Could you check a few things on this model? Use its own coordinates, in mm. A direction names the side the tool comes from. Give positions to 0.01 mm unless a question says otherwise; leave off trailing zeros. Loops run counter-clockwise (first coordinate to the right, second up) from the corner with the lowest first, then second, coordinate; pieces in that order, holes last. Notation, with made-up numbers: M 68,16.5 L 75,16.5 A29 cw 75,50.5 Z; hole C 24,47.25 d10. An arc over 180 degrees is marked long. Use CSV: the item, a comma, the result in double quotes.
```python
from build123d import *

# Parameters (mm, degrees)
SKETCH1_W            = 195
SKETCH1_H            = 145
BOSS_EXTRUDE1_DEPTH  = 5
SKETCH2_W            = 63.6
SKETCH2_H            = 2
SKETCH2_W_2          = 63.5
BOSS_EXTRUDE2_DEPTH  = 9.5
SKETCH4_W            = 8
SKETCH4_H            = 8
BOSS_EXTRUDE3_DEPTH  = 30
SKETCH3_W            = 2
SKETCH3_H            = 19
BOSS_EXTRUDE11_DEPTH = 12.6
SKETCH8_W            = 14
SKETCH8_H            = 14
SKETCH8_W_2          = 8
SKETCH8_H_2          = 8
BOSS_EXTRUDE12_DEPTH = 2
FILLET2_R            = 10
FILLET3_R            = 3


with BuildPart() as part:
    # Sketch1 → Boss-Extrude1 (new body)
    with BuildSketch(Plane(origin=(0, 0, 0), x_dir=(1, 0, 0), z_dir=(0, 1, 0))):
        Rectangle(SKETCH1_W, SKETCH1_H)
    extrude(amount=BOSS_EXTRUDE1_DEPTH)

    # Sketch2 → Boss-Extrude2 (add)
    with BuildSketch(Plane(origin=(0, 5, 0), x_dir=(1, 0, 0), z_dir=(0, 1, 0))):
        Polygon((-82.5, -57.5), (-82.5, -3.6), (-70, -3.6), (-70, -1.6), (-84.5, -1.6), (-84.5, -59.5), (84.5, -59.5), (84.5, -1.6), (70, -1.6), (70, -3.6), (82.5, -3.6), (82.5, -57.5), align=None)
        with Locations((-33.9, -2.6)):
            Rectangle(SKETCH2_W, SKETCH2_H)
        with Locations((33.95, -2.6)):
            Rectangle(SKETCH2_W_2, SKETCH2_H)
    extrude(amount=BOSS_EXTRUDE2_DEPTH)

    # Sketch4 → Boss-Extrude3 (add)
    with BuildSketch(Plane(origin=(0, 5, 0), x_dir=(1, 0, 0), z_dir=(0, 1, 0))):
        with Locations((-90.5, -65.5)):
            Rectangle(SKETCH4_W, SKETCH4_H)
        with Locations((90.5, -65.5)):
            Rectangle(SKETCH4_W, SKETCH4_H)
        with Locations((90.5, 65.5)):
            Rectangle(SKETCH4_W, SKETCH4_H)
        with Locations((-90.5, 65.5)):
            Rectangle(SKETCH4_W, SKETCH4_H)
    extrude(amount=BOSS_EXTRUDE3_DEPTH)

    # Sketch3 → Boss-Extrude11 (add)
    with BuildSketch(Plane(origin=(0, 5, 0), x_dir=(1, 0, 0), z_dir=(0, 1, 0))):
        with Locations((-52.2, 26.9)):
            Rectangle(SKETCH3_W, SKETCH3_H)
        Polygon((-51.2, 48.5), (-51.2, 57.5), (51.2, 57.5), (51.2, 4.4), (-51.2, 4.4), (-51.2, 8.4), (-53.2, 8.4), (-53.2, 2.4), (53.2, 2.4), (53.2, 59.5), (-53.2, 59.5), (-53.2, 48.5), align=None)
    extrude(amount=BOSS_EXTRUDE11_DEPTH)

    # Sketch8 → Boss-Extrude12 (add)
    with BuildSketch(Plane(origin=(0, 30, 0), x_dir=(1, 0, 0), z_dir=(0, 1, 0))):
        with Locations((90.5, 65.5)):
            Rectangle(SKETCH8_W, SKETCH8_H)
        with Locations((90.5, 65.5)):
            Rectangle(SKETCH8_W_2, SKETCH8_H_2, mode=Mode.SUBTRACT)
        with Locations((90.5, -65.5)):
            Rectangle(SKETCH8_W, SKETCH8_H)
        with Locations((90.5, -65.5)):
            Rectangle(SKETCH8_W_2, SKETCH8_H_2, mode=Mode.SUBTRACT)
        with Locations((-90.5, -65.5)):
            Rectangle(SKETCH8_W, SKETCH8_H)
        with Locations((-90.5, -65.5)):
            Rectangle(SKETCH8_W_2, SKETCH8_H_2, mode=Mode.SUBTRACT)
        with Locations((-90.5, 65.5)):
            Rectangle(SKETCH8_W, SKETCH8_H)
        with Locations((-90.5, 65.5)):
            Rectangle(SKETCH8_W_2, SKETCH8_H_2, mode=Mode.SUBTRACT)
    extrude(amount=-BOSS_EXTRUDE12_DEPTH)

    # Fillet2
    fillet2_edges = [part.edges().sort_by_distance(p)[0] for p in [
        (-97.5, 2.5, -72.5),
        (97.5, 2.5, -72.5),
        (97.5, 2.5, 72.5),
        (-97.5, 2.5, 72.5),
    ]]
    fillet(fillet2_edges, radius=FILLET2_R)

    # Fillet3
    fillet3_edges = [part.edges().sort_by_distance(p)[0] for p in [
        (97.5, 29, -58.5),
        (83.5, 29, -58.5),
        (83.5, 29, -72.5),
        (97.5, 29, -72.5),
        (83.5, 29, 58.5),
        (97.5, 29, 58.5),
        (97.5, 29, 72.5),
        (83.5, 29, 72.5),
        (-97.5, 29, 58.5),
        (-83.5, 29, 58.5),
        (-83.5, 29, 72.5),
        (-97.5, 29, 72.5),
        (-83.5, 29, -58.5),
        (-97.5, 29, -58.5),
        (-97.5, 29, -72.5),
        (-83.5, 29, -72.5),
    ]]
    fillet(fillet3_edges, radius=FILLET3_R)


solid = part.part
```
1. I want a section at C-C, the plane x = -19. List the corners of the cut face in (y, z) for me, then the cut area to 3 significant figures.
Outcome:
outline,"M 0,-72.5 L 5,-72.5 L 5,-59.5 L 17.6,-59.5 L 17.6,-57.5 L 5,-57.5 L 5,-4.4 L 17.6,-4.4 L 17.6,-2.4 L 5,-2.4 L 5,1.6 L 14.5,1.6 L 14.5,3.6 L 5,3.6 L 5,57.5 L 14.5,57.5 L 14.5,59.5 L 5,59.5 L 5,72.5 L 0,72.5 Z"
area,"813 mm2"
2. Which directions (+Z, -Z, +X, -X, +Y, -Y) give clear straight access to the entire face, cutting with the end or side of a thin tool? Please do faces 5 (the face through (-53.2, 11, -54)), 6 (the face through (-51.2, 11, -53)), 7 (the face through (-94.5, 16, 66)), 8 (the face through (-77, 10, 1.6)), 9 (the face through (94.49, 2.54, -69.65)).
Outcome:
face 5,"-Z, -X, +Y"
face 6,"+Y"
face 7,"+Z, -Z, -X"
face 8,"-Z, +X, -X, +Y"
face 9,"-Z, +X, -Y"
3. I want a section at B-B, the plane z = -24.5. List the corners of the cut face in (x, y) for me, then the cut area to 3 significant figures.
Outcome:
outline,"M -97.5,0 L 97.5,0 L 97.5,5 L 53.2,5 L 53.2,17.6 L 51.2,17.6 L 51.2,5 L -51.2,5 L -51.2,17.6 L -53.2,17.6 L -53.2,5 L -97.5,5 Z"
area,"1,030 mm2"
4. I'm going to push flat-ended pins straight in: pin 1 Ø3 at (x, y) = (47.5, 8.5) entering from +Z; pin 2 Ø12 at (x, y) = (-40.5, 17) entering from -Z; pin 3 Ø4 at (x, y) = (90.5, 33.5) entering from +Z. Where does each tip first touch, or does it pass through?
Outcome:
pin 1,"z = 59.5"
pin 2,"z = -59.5"
pin 3,"z = 69.5"
5. I want a section at D-D, the plane z = 26. List the corners of the cut face in (x, y) for me, then the cut area to 3 significant figures.
Outcome:
outline,"M -97.5,0 L 97.5,0 L 97.5,5 L 84.5,5 L 84.5,14.5 L 82.5,14.5 L 82.5,5 L -82.5,5 L -82.5,14.5 L -84.5,14.5 L -84.5,5 L -97.5,5 Z"
area,"1,010 mm2"
6. If we mould it in two halves opening along X, with no side actions, what happens to faces 1 (the face through (94.5, 32, 66)), 2 (the face through (90, 30, -70)), 3 (the face through (90, 35, 65)), 4 (the face through (-86, 30, -66))? For each: +X half, -X half, draft (parallel to the pull), parting line (faces both ways), or undercut.
Outcome:
face 1,"+X half"
face 2,"undercut"
face 3,"draft"
face 4,"undercut"
7. I want a section at A-A, the plane y = 24. List the corners of the cut face in (x, z) for me, then the cut area to 3 significant figures.
Outcome:
outline,"M -94.5,-69.5 L -86.5,-69.5 L -86.5,-61.5 L -94.5,-61.5 Z; M -94.5,61.5 L -86.5,61.5 L -86.5,69.5 L -94.5,69.5 Z; M 86.5,-69.5 L 94.5,-69.5 L 94.5,-61.5 L 86.5,-61.5 Z; M 86.5,61.5 L 94.5,61.5 L 94.5,69.5 L 86.5,69.5 Z"
area,"256 mm2"
8. Please list where these lines run through material, in increasing order: line 1 (Z direction, x = 28.5, y = 8); line 2 (X direction, y = 15, z = -23.5); line 3 (X direction, y = 7.5, z = 47.5).
Outcome:
line 1,"-59.5 to -57.5, -4.4 to -2.4, 1.6 to 3.6, 57.5 to 59.5"
line 2,"-53.2 to -51.2, 51.2 to 53.2"
line 3,"-84.5 to -82.5, 82.5 to 84.5"
